Verification items for the finished model (mm, model axes). A direction names the side the tool comes from. Coordinates: 2 decimals unless noted, no trailing zeros. Write each loop counter-clockwise with the first axis right and the second up, starting at its lowest first coordinate (ties: lowest second). Pieces come first, ordered by that corner, then holes.
Autodesk Inventor part; units mm, degrees
ref_plane "YZ Plane" through (0, 0, 0) normal (1, 0, 0) x (0, 1, 0)
ref_plane "XZ Plane" through (0, 0, 0) normal (0, 1, 0) x (-1, 0, 0)
ref_plane "XY Plane" through (0, 0, 0) normal (0, 0, 1) x (1, 0, 0)
sketch "Sketch1" plane through (0, 0, 0) normal (0, 0, 1) x (1, 0, 0)
  arc A0 (6.1036, -1.9996) -> (-16.8874, -1.4338) centre (-5.2593, 3.6728) ccw
  arc A1 (1.5584, 0.2694) -> (-12.2361, 0.6088) centre (-5.2593, 3.6728) ccw
  line L0 (-12.2361, 0.6088) -> (-16.8874, -1.4338)
  line L1 (1.5584, 0.2694) -> (6.1036, -1.9996)
  point P0 (0, 0)
  dimension "d0" = 25.4
  dimension "d1" = 15.24
extrude "Extrusion1" add sketch "Sketch1" along normal blind 25.4
sketch "Sketch2" plane through (0, 0, 25.4) normal (0, 0, 1) x (1, 0, 0)
  arc A0 (6.1036, -1.9996) -> (-16.8874, -1.4338) centre (-5.2593, 3.6728) ccw
  line L0 (-5.2593, 16.3728) -> (1.9559, 16.3728) construction
  arc A1 (1.5584, 0.2694) -> (-12.2361, 0.6088) centre (-5.2593, 3.6728) ccw
  line L1 (-5.2593, 11.2928) -> (0.7923, 11.2928) construction
  point P0 (0, 0)
  point P1 (-12.1004, 0.3168)
  point P2 (1.2826, -0.2347)
ref_plane "Work Plane2" through (-5.2593, 11.2928, 25.4) normal (0, -1, 0) x (1, 0, 0)
sketch "Sketch3" plane through (-5.2593, 11.2928, 25.4) normal (0, -1, 0) x (1, 0, 0)
  line L0 (12.7, 0) -> (-12.7, 0)
  line L1 (-12.7, -25.4) -> (12.7, -25.4)
  line L2 (-12.7, 0) -> (12.7, -25.4) construction
  line L3 (12.7, 0) -> (-12.7, -25.4) construction
  circle A0 centre (0, -12.7) radius 8.89
  point P0 (5.2593, -25.4)
  point P1 (11.3628, 0)
  point P2 (-11.6281, 0)
  point P3 (11.3628, -25.4)
  point P4 (-11.6281, -25.4)
  dimension "d4" = 17.78
extrude "Extrusion2" add sketch "Sketch3" against normal blind 127
properties part number "golf1"
1. Material ranges on L1, parallel to Y at x = -5.75, z = 1.5; L2, parallel to X at y = 10, z = 18.5; L3, parallel to Y at x = -14.5, z = 9.75, recorded low to high.
2. Sectioned sample at D-D, the plane y = 84.5. Record the boundary of the cut face in (x, z), and give its area (3 significant figures).
3. Sectioned sample at A-A, the plane y = 9. Record the boundary of the cut face in (x, z).
4. Tool access check on faces 4 (the flat face through (-5, 138.293, 13)), 5 (the cylindrical face through (-0.48, 74.638, 20.196)), 6 (the flat face through (3.8, -0.85, 12.52)). Record the directions out of +Z, -Z, +X, -X, +Y, -Y that give a thin tool (end or side, any length) a straight path to the whole face; none if there is none.
5. Sectioned sample at C-C, the plane z = 20.25. Record the boundary of the cut face in (x, y).
6. Sectioned sample at B-B, the plane x = -1.25. Record the boundary of the cut face in (y, z), and give its area (3 significant figures).
7. Gauge pin test, flat ends, axial feed: P1, Ø12, axis at y = 30.5, z = 22.5, coming from the -X side; P2, Ø3, axis at x = -15, z = 21, coming from the +Y side; P3, Ø8, axis at x = 3, y = 113, coming from the -Z side. Record the tip position at first contact, or that the pin passes through.
8. Draft check along X on faces 1 (the cylindrical face through (4.605, 11.672, 12.522)), 2 (the flat face through (-14.53, -0.4, 12.52)), 3 (the flat face through (-2.6, 11.4, 25.4)). Enter one of: pulls with the +X half, pulls with the -X half, needs draft (parallel to the pull), parting line crosses it, or undercut.
Outcome:
1. L1: y = 11.28 to 16.36
1. L2: x = -16.27 to -9.51, -1.01 to 5.75
1. L3: y = -0.39 to 12.38
2. outline: circle Ø17.78 at (-5.26, 12.7)
2. area: 248 mm2
3. outline: (-16.79, 0) - (-10.71, 0) - (-10.71, 25.4) - (-16.79, 25.4) - close; (0.19, 0) - (6.27, 0) - (6.27, 25.4) - (0.19, 25.4) - close
4. face 4: +Z, -Z, +X, -X, +Y
4. face 5: +Y
4. face 6: +Z, -Z, -Y
5. outline: (-16.89, -1.43) - (-12.24, 0.61) arc R7.62 cw (long way) to (1.56, 0.27) - (6.1, -2) arc R12.7 ccw to (-0.57, 15.47) - (-0.57, 138.29) - (-9.95, 138.29) - (-9.95, 15.47) arc R12.7 ccw to start
6. outline: (10.15, 0) - (15.72, 0) - (15.72, 4.77) - (138.29, 4.77) - (138.29, 20.63) - (15.72, 20.63) - (15.72, 25.4) - (10.15, 25.4) - close
6. area: 2,090 mm2
7. P1: stops at x = -13.3
7. P2: stops at y = 13.34
7. P3: stops at z = 4.9
8. face 1: parting line crosses it
8. face 2: undercut
8. face 3: needs draft
